Read the model definition and answer for the solid it produces. Units are mm, in the model's axes. Give positions to 0.01 mm unless a question says otherwise; leave off trailing zeros. Order: outer loops, then holes, each group sorted by start corner. A loop starts at its lowest first (then second) coordinate and runs counter-clockwise, first axis right, second up. Notation, with made-up numbers: (59, -20.5) - (63, -20.5) arc R16 cw to (63, 7.5) - close; hole circle Ø9 at (41, 48). An arc over 180 degrees is marked (long way). Return JSON: item names as keys, results as strings.
Autodesk Inventor part; units mm, degrees
ref_plane "YZ Plane" through (0, 0, 0) normal (1, 0, 0) x (0, 1, 0)
ref_plane "XZ Plane" through (0, 0, 0) normal (0, 1, 0) x (-1, 0, 0)
ref_plane "XY Plane" through (0, 0, 0) normal (0, 0, 1) x (1, 0, 0)
sketch "Sketch1" plane through (0, 0, 0) normal (0, 0, 1) x (1, 0, 0)
  circle A0 centre (0, 0) radius 8.7313
  circle A1 centre (0, 0) radius 11.1125
  circle A2 centre (0, 0) radius 3.175
  dimension "d0" = 17.4625
  dimension "d1" = 22.225
  dimension "d2" = 6.35
extrude "Extrusion1" add sketch "Sketch1" along normal blind 6.35 contours A0
extrude "Extrusion2" add sketch "Sketch1" against normal blind 1.5875 contours A0 | A1
chamfer "Chamfer1" distance 0.254 angle 45 5 edges at (-8.7313, 0, 6.35) (-11.1125, 0, 0) (-11.1125, 0, -1.5875) (-3.175, 0, 6.35) (-3.175, 0, -1.5875)
properties part number "0.25 in Flanged Ball Bearing" material "Steel"
Q1. Consider L1, parallel to Y at x = 0, z = 2.75 (3 decimals); L2, parallel to Y at x = -1, z = 2; L3, parallel to X at y = 0.5, z = 0.5. Determine where each line is inside the solid, lowest interval first.
Values:
{"L1": "y = -8.731 to -3.175, 3.175 to 8.731", "L2": "y = -8.67 to -3.01, 3.01 to 8.67", "L3": "x = -8.72 to -3.14, 3.14 to 8.72"}
Q2. Given pin 1 (3 mm diameter, centred on y = -3, z = 3.5, fed in from -X); pin 2 (5 mm diameter, centred on x = 0, y = 0, fed in from -Z); pin 3 (3 mm diameter, centred on y = 7, z = 5, fed in from -X), each flat-ended and moving along its own axis, determine where each tip first touches the part or whether it passes through.
Values:
{"pin 1": "stops at x = -8.6", "pin 2": "passes through", "pin 3": "stops at x = -6.78"}
Q3. A cutting plane is placed at C-C (z = 3). Write down the section's boundary in (x, y) (3 decimals).
Values:
{"outline": "circle Ø17.463 at (0, 0); hole circle Ø6.35 at (0, 0)"}
Q4. Determine the mould class of faces 1 (the flat face through (1, 9, 0)), 2 (the cylindrical face through (-6.93, 5.31, 3.01)), 3 (the cylindrical face through (-0.69, 3.1, 2.33)) for opening direction X: released by +X, released by -X, zero draft, split by the parting line, or undercut.
Values:
{"face 1": "zero draft", "face 2": "split by the parting line", "face 3": "undercut"}
